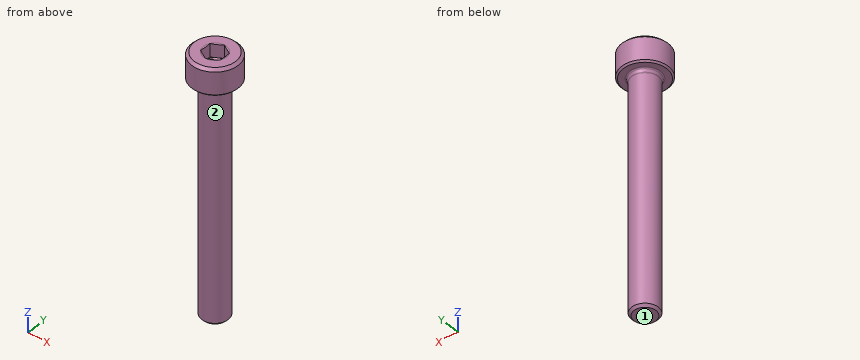
```python
from build123d import *

# Parameters (mm, degrees)
CUT_EXTRUDE1_DEPTH = 2


with BuildPart() as part:
    # Sketch1 → Revolve1 (revolve)
    with BuildSketch(Plane(origin=(0, 0, 0), x_dir=(0, 0, -1), z_dir=(1, 0, 0))):
        with BuildLine():
            Line((0, 0), (0, 3.1))
            Line((0, 3.1), (0.4, 3.5))
            Line((0.4, 3.5), (3.765, 3.5))
            Line((3.765, 3.5), (4, 3.265))
            Line((4, 3.265), (4, 2.35))
            ThreePointArc((4, 2.35), (4.035614876, 2.236081032), (4.129775312, 2.162734164))
            Line((4.129775312, 2.162734164), (4.529775312, 2.012734164))
            ThreePointArc((4.529775312, 2.012734164), (4.564315039, 2.00320929), (4.6, 2))
            Line((4.6, 2), (38.65, 2))
            Line((38.65, 2), (39, 1.65))
            Line((39, 1.65), (39, 0))
            Line((39, 0), (0, 0))
        make_face()
    revolve(axis=Axis((0, 0, 0), (0, 0, -1)))

    # Sketch2 → Cut-Extrude1 (cut)
    with BuildSketch(Plane.XY):
        Polygon((0, 1.732050808), (-1.5, 0.866025404), (-1.5, -0.866025404), (0, -1.732050808), (1.5, -0.866025404), (1.5, 0.866025404), align=None)
    extrude(amount=-CUT_EXTRUDE1_DEPTH, mode=Mode.SUBTRACT)

    # Sketch3 → Cut-Revolve2 (revolve, cut)
    with BuildSketch(Plane(origin=(0, 0, 0), x_dir=(0, 0, -1), z_dir=(1, 0, 0))):
        Polygon((2, 0), (2, 1.5), (2.866025404, 0), align=None)
    revolve(axis=Axis((0, 0, -2), (0, 0, -1)), mode=Mode.SUBTRACT)

    # Sketch4 → Cut-Revolve3 (revolve, cut)
    with BuildSketch(Plane(origin=(0, 0, 0), x_dir=(0, 0, -1), z_dir=(1, 0, 0))):
        Polygon((0, 1.732050808), (0, 1.5), (0.062177826, 1.5), align=None)
    revolve(axis=Axis((0, 0, 0), (0, 0, -1)), mode=Mode.SUBTRACT)


solid = part.part
```
The listing builds one solid part. Answer for the finished solid, in the listing's coordinates (mm). Face numbers are marked on the shaded views. A direction names the side the tool comes from. Round coordinates to 2 decimals unless told otherwise and drop trailing zeros. Loops run counter-clockwise (first coordinate to the right, second up) from the corner with the lowest first, then second, coordinate; pieces in that order, holes last. Notation, with made-up numbers: (69.25, -30) - (119.25, -30) arc R12 ccw to (119.25, -10) - close; hole circle Ø11 at (-13.5, 4). An arc over 180 degrees is marked (long way). Use one line per item in the form item = value. Start each with the question number.
1. The part is cut by section A-A on z = -22.5. Determine the outline of the cut face in (x, y).
2. Given pin 1 Ø2 at (y, z) = (2.5, -23.5) entering from +X; pin 2 Ø3 at (x, z) = (-2.5, -22.5) entering from -Y; pin 3 Ø0.5 at (x, y) = (0, -1.5) entering from +Z; pin 4 Ø3 at (y, z) = (2.5, -23) entering from -X, each flat-ended and moving along its own axis, determine where each tip first touches the part or whether it passes through.
3. A tool of negligible diameter and unlimited length cuts with its end or side. For the marked faces 1 and 2, from which of +Z, -Z, +X, -X, +Y, -Y can it reach the whole face along a straight path? Write none if from no direction.
4. Consider line 1 (Z direction, x = 0.5, y = 2.75); line 2 (X direction, y = -1, z = -32); line 3 (X direction, y = 0, z = -29). Determine where each line is inside the solid, lowest interval first. Write a range as [from, to].
Geometry check:
q1.outline = circle Ø4 at (0, 0)
q2.pin_1 = 1.32
q2.pin_2 = -1.73
q2.pin_3 = 0
q2.pin_4 = -1.73
q3.face_1 = -Z, +X, -X, +Y, -Y
q3.face_2 = -Z
q4.line_1 = [-4, 0]
q4.line_2 = [-1.73, 1.73]
q4.line_3 = [-2, 2]
